from build123d import *

# Parameters (mm, degrees)
SKETCH1_R           = 31.75
BOSS_EXTRUDE1_DEPTH = 160.1978
SKETCH2_R           = 25.4
BOSS_EXTRUDE2_DEPTH = 57.15
BOSS_EXTRUDE3_START = 57.15
SKETCH3_R           = 25.4
BOSS_EXTRUDE3_DEPTH = 57.15
SKETCH5_R           = 17.4625
BOSS_EXTRUDE5_DEPTH = 25.4
BOSS_EXTRUDE6_START = 57.15
SKETCH18_R          = 17.4625
BOSS_EXTRUDE6_DEPTH = 57.15
SKETCH20_W          = 7.9248
SKETCH20_H          = 7.9248
CUT_EXTRUDE1_DEPTH  = 44.45


with BuildPart() as part:
    # Sketch1 → Boss-Extrude1 (new, symmetric)
    with BuildSketch(Plane.XY):
        with Locations(Location((0, 0, 0), (0, 0, 180))):
            Circle(SKETCH1_R)
    extrude(amount=BOSS_EXTRUDE1_DEPTH, both=True)

    # Sketch2 → Boss-Extrude2 (add)
    with BuildSketch(Plane.XY.offset(160.1978)):
        Circle(SKETCH2_R)
    extrude(amount=BOSS_EXTRUDE2_DEPTH)

    # Sketch3 → Boss-Extrude3 (add)
    with BuildSketch(Plane(origin=(0, 0, -160.1978), x_dir=(-1, 0, 0), z_dir=(0, 0, -1)).offset(BOSS_EXTRUDE3_START)):
        with Locations(Location((0, 0, 0), (0, 0, 180))):
            Circle(SKETCH3_R)
    extrude(amount=-BOSS_EXTRUDE3_DEPTH)

    # Sketch5 → Boss-Extrude5 (add)
    with BuildSketch(Plane(origin=(0, 0, -217.3478), x_dir=(-1, 0, 0), z_dir=(0, 0, -1))):
        Circle(SKETCH5_R)
    extrude(amount=BOSS_EXTRUDE5_DEPTH)

    # Sketch18 → Boss-Extrude6 (add)
    with BuildSketch(Plane.XY.offset(217.3478).offset(BOSS_EXTRUDE6_START)):
        with Locations(Location((0, 0, 0), (0, 0, 180))):
            Circle(SKETCH18_R)
    extrude(amount=-BOSS_EXTRUDE6_DEPTH)

    # Sketch20 → Cut-Extrude1 (cut)
    with BuildSketch(Plane.XY.offset(274.4978)):
        with Locations((0, 17.4625)):
            Rectangle(SKETCH20_W, SKETCH20_H)
    extrude(amount=-CUT_EXTRUDE1_DEPTH, mode=Mode.SUBTRACT)


solid = part.part
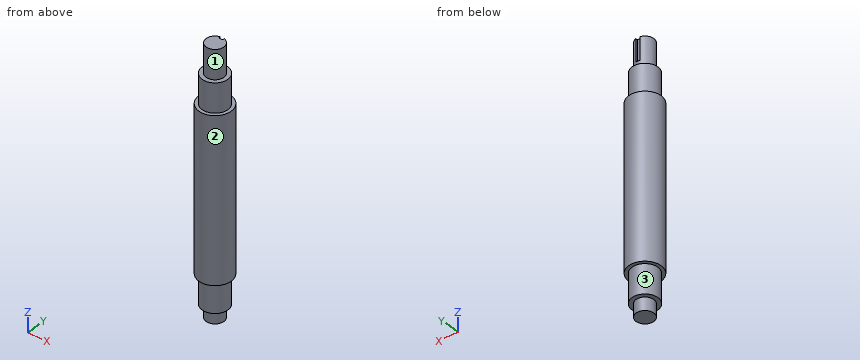
Input: part model. Units: mm. Frame: model coordinates. Face numbers are marked on the shaded views. A direction names the side the tool comes from. Round coordinates to 2 decimals unless told otherwise and drop trailing zeros. Order: outer loops, then holes, each group sorted by start corner. A loop starts at its lowest first (then second) coordinate and runs counter-clockwise, first axis right, second up. Notation, with made-up numbers: (-24, -37) - (-18, -37) arc R13 cw to (-18, -15) - close; hole circle Ø4 at (-6.75, -23.5). An arc over 180 degrees is marked (long way). Use a Markdown table: item, result.
1. Section C-C on z = 127. Return the cut outline in (x, y).
Evaluation:
| item | result |
|---|---|
| outline | circle Ø63.5 at (0, 0) |
2. Material intervals for probe 1 along Z at (x, y) = (-24.5, 10); probe 2 along Z at (x, y) = (-15, 9); probe 3 along X at (y, z) = (18.5, -105), sorted ascending.
Evaluation:
| item | result |
|---|---|
| probe 1 | -160.2 to 160.2 |
| probe 2 | -217.35 to 217.35 |
| probe 3 | -25.8 to 25.8 |
3. First-contact query: pin 1 (1 mm diameter, centred on x = 13.5, z = 173, fed in from +Y); pin 2 (2 mm diameter, centred on x = 7.5, z = 61, fed in from -Y); pin 3 (5 mm diameter, centred on x = 13, z = -43.5, fed in from +Y). Flat tips, straight axial feed; report the tip coordinate or a pass-through.
Evaluation:
| item | result |
|---|---|
| pin 1 | y = 21.82 |
| pin 2 | y = -31.08 |
| pin 3 | y = 29.96 |
4. Access query for the marked faces 1, 2 and 3. Directions: +Z, -Z, +X, -X, +Y, -Y. A direction counts if a zero-diameter tool reaches every point of the face in a straight line with its end or side. Return the directions, or none.
Evaluation:
| item | result |
|---|---|
| face 1 | +Z |
| face 2 | +Z, -Z |
| face 3 | -Z |
5. Section B-B on z = 238. Return the cut outline in (x, y) (1 decimal), then the cut area to 3 significant figures.
Evaluation:
| item | result |
|---|---|
| outline | (-4, 13.5) - (-4, 17) arc R17.5 ccw (long way) to (4, 17) - (4, 13.5) - close |
| area | 928 mm^2 |
6. Section D-D on z = 181.5. Return the cut outline in (x, y).
Evaluation:
| item | result |
|---|---|
| outline | circle Ø50.8 at (0, 0) |
7. Section A-A on y = 0. Return the cut outline in (x, z), then the cut area to 3 significant figures.
Evaluation:
| item | result |
|---|---|
| outline | (-31.75, -160.2) - (-25.4, -160.2) - (-25.4, -217.35) - (-17.46, -217.35) - (-17.46, -242.75) - (17.46, -242.75) - (17.46, -217.35) - (25.4, -217.35) - (25.4, -160.2) - (31.75, -160.2) - (31.75, 160.2) - (25.4, 160.2) - (25.4, 217.35) - (17.46, 217.35) - (17.46, 274.5) - (-17.46, 274.5) - (-17.46, 217.35) - (-25.4, 217.35) - (-25.4, 160.2) - (-31.75, 160.2) - close |
| area | 29,000 mm^2 |
